The listing builds one solid part. Answer for the finished solid, in the listing's coordinates (mm). Face numbers are marked on the shaded views. A direction names the side the tool comes from. Round coordinates to 2 decimals unless told otherwise and drop trailing zeros. Write each loop counter-clockwise with the first axis right and the second up, starting at its lowest first coordinate (ties: lowest second). Pieces come first, ordered by that corner, then holes.
Autodesk Inventor part; units mm, degrees
ref_plane "YZ Plane" through (0, 0, 0) normal (1, 0, 0) x (0, 1, 0)
ref_plane "XZ Plane" through (0, 0, 0) normal (0, 1, 0) x (-1, 0, 0)
ref_plane "XY Plane" through (0, 0, 0) normal (0, 0, 1) x (1, 0, 0)
sketch "Sketch1" plane through (0, 0, 0) normal (1, 0, 0) x (0, 1, 0)
  line L0 (0, 0) -> (0, -25)
  line L1 (0, -25) -> (3, -25)
  line L2 (3, -25) -> (1.5, -23.5)
  line L3 (1.5, -23.5) -> (1.5, 0)
  line L4 (1.5, 0) -> (0, 0)
  dimension "d0" = 6
  dimension "d1" = 25
  dimension "d2" = 45
  dimension "d3" = 3
revolve "Revolution1" add sketch "Sketch1" angle 360 about axis through (0, 0, 0) along (0, 0, -1)
chamfer "Chamfer1" distance 0.2 angle 45 1 edges at (0, -1.5, 0)
thread "Thread1"
sketch "Sketch2" plane through (0, 0, -25) normal (0, 0, -1) x (-1, 0, 0)
  circle A0 centre (0, 0) radius 1.3
  line L0 (1.1547, 0) -> (0.5774, -1)
  line L1 (0.5774, -1) -> (-0.5774, -1)
  line L2 (-0.5774, -1) -> (-1.1547, 0)
  line L3 (-1.1547, 0) -> (-0.5774, 1)
  line L4 (-0.5774, 1) -> (0.5774, 1)
  line L5 (0.5774, 1) -> (1.1547, 0)
  dimension "d10" = 2
extrude "Extrusion1" cut sketch "Sketch2" against normal blind 1.2 contours L0 L1 L2 L3 L4 L5
properties part number "M3 x 25 mm FHCS"
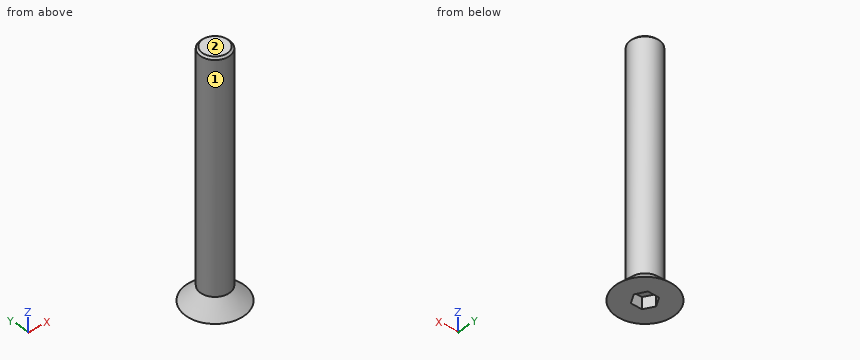
1. Straight lines are drawn through the part: line 1 along X through (y, z) = (0, -1.25); line 2 along X through (y, z) = (-0.75, -20); line 3 along Z through (x, y) = (2.3, -0.05). For each, find the intervals that lie inside material, in ascending order.
Geometry says:
line 1: x = -1.5 to 1.5
line 2: x = -1.3 to 1.3
line 3: z = -25 to -24.3
2. Section B-B on z = -19.5 is taken. Determine the outline of the cut face in (x, y).
Geometry says:
outline: circle Ø3 at (0, 0)
3. A tool of negligible diameter and unlimited length cuts with its end or side. For the marked faces 1 and 2, from which of +Z, -Z, +X, -X, +Y, -Y can it reach the whole face along a straight path? Write none if from no direction.
Geometry says:
face 1: +Z
face 2: +Z, +X, -X, +Y, -Y
4. Section A-A on x = 0 is taken. Determine the outline of the cut face in (y, z).
Geometry says:
outline: (-3, -25) - (-1, -25) - (-1, -23.8) - (1, -23.8) - (1, -25) - (3, -25) - (1.5, -23.5) - (1.5, -0.2) - (1.3, 0) - (-1.3, 0) - (-1.5, -0.2) - (-1.5, -23.5) - close
5. Given pin 1 (1 mm diameter, centred on x = -0.5, y = 0, fed in from -Z); pin 2 (0.9 mm diameter, centred on x = 0.5, z = -24, fed in from +Y); pin 3 (1 mm diameter, centred on x = 0, y = 2, fed in from +Z), each flat-ended and moving along its own axis, determine where each tip first touches the part or whether it passes through.
Geometry says:
pin 1: stops at z = -23.8
pin 2: stops at y = 2.41
pin 3: stops at z = -23.5
